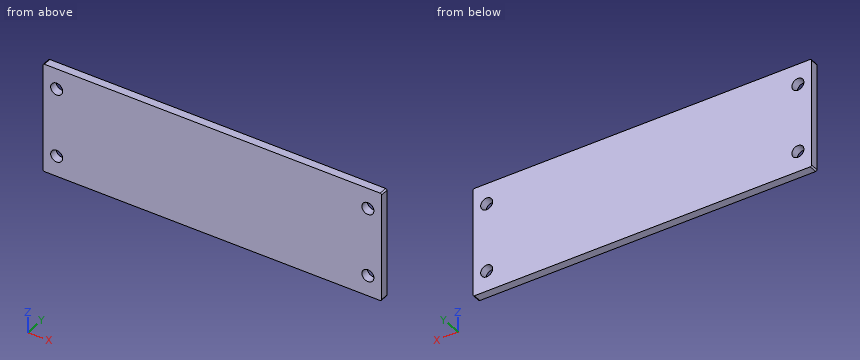
Autodesk Fusion 360 part; units mm, degrees
sketch "Sketch1" plane through (0, 0, 0) normal (0, 1, 0) x (1, 0, 0)
  line L0 (-61.5, -20) -> (61.5, -20)
  line L1 (62, -19.5) -> (62, 19.5)
  line L2 (61.5, 20) -> (-61.5, 20)
  line L3 (-62, 19.5) -> (-62, -19.5)
  line L4 (-62, -20) -> (62, 20) construction
  line L5 (62, -20) -> (-62, 20) construction
  line L6 (62, 20) -> (57, 20)
  line L7 (57, 20) -> (57, 12.5) construction
  line L8 (57, 12.5) -> (62, 12.5) construction
  line L9 (62, 12.5) -> (62, 20)
  line L10 (62, -20) -> (57, -20)
  line L11 (57, -20) -> (57, -12.5) construction
  line L12 (57, -12.5) -> (62, -12.5) construction
  line L13 (62, -12.5) -> (62, -20)
  line L14 (-62, -20) -> (-57, -20)
  line L15 (-57, -20) -> (-57, -12.5) construction
  line L16 (-57, -12.5) -> (-62, -12.5) construction
  line L17 (-62, -12.5) -> (-62, -20)
  line L18 (-62, 20) -> (-57, 20)
  line L19 (-57, 20) -> (-57, 12.5) construction
  line L20 (-57, 12.5) -> (-62, 12.5) construction
  line L21 (-62, 12.5) -> (-62, 20)
  circle A0 centre (57, -12.5) radius 2.2
  circle A1 centre (-57, -12.5) radius 2.2
  circle A2 centre (57, 12.5) radius 2.2
  circle A3 centre (-57, 12.5) radius 2.2
  arc A4 (61.5, -20) -> (62, -19.5) centre (61.5, -19.5) ccw
  arc A5 (-62, -19.5) -> (-61.5, -20) centre (-61.5, -19.5) ccw
  arc A6 (-61.5, 20) -> (-62, 19.5) centre (-61.5, 19.5) ccw
  arc A7 (62, 19.5) -> (61.5, 20) centre (61.5, 19.5) ccw
  dimension "d1" = 124
  dimension "d2" = 40
  dimension "d3" = 5
  dimension "d4" = 7.5
  dimension "d5" = 5
  dimension "d6" = 7.5
  dimension "d7" = 5
  dimension "d8" = 7.5
  dimension "d9" = 5
  dimension "d10" = 7.5
  dimension "d11" = 4.4
  dimension "d12" = 4.4
  dimension "d13" = 4.4
  dimension "d14" = 4.4
  dimension "d15" = 0.5
extrude "Extrude1" add sketch "Sketch1" along normal blind 3 contours L0 L1 L2 L3 L6 L9 L10 L13 L14 L17 L18 L21 A4 A5 A6 A7
For this review, take the finished solid that the model builds, in its own axes (mm). Give positions to 0.01 mm unless a question says otherwise; leave off trailing zeros. Loops run counter-clockwise (first coordinate to the right, second up) from the corner with the lowest first, then second, coordinate; pieces in that order, holes last. Notation, with made-up numbers: M -34,18.25 L 3,18.25 A24 cw 3,44.25 Z; hole C 0.25,39 d8. An arc over 180 degrees is marked long. Answer as a JSON object with one key per item and string values. Group by question number.
Q1. Add section A-A on x = 57. Give the boundary of the cut face in (y, z), and give its area (3 significant figures).
Q2. For probe 1 along X at (y, z) = (1.85, -12.5); probe 2 along Z at (x, y) = (-57, 2.05); probe 3 along X at (y, z) = (0.1, 13), list the stretches that pass through material, from the lowest coordinate up. Write a range as [from, to].
Q3. Add section B-B on z = -12.5. Give the boundary of the cut face in (x, y), and give its area (3 significant figures).
Checked values:
{
 "1": {"outline": "M 0,-20 L 3,-20 L 3,-14.7 L 0,-14.7 Z; M 0,-10.3 L 3,-10.3 L 3,10.3 L 0,10.3 Z; M 0,14.7 L 3,14.7 L 3,20 L 0,20 Z", "area": "93.6 mm²"},
 "2": {"probe 1": "[-62, -59.2], [-54.8, 54.8], [59.2, 62]", "probe 2": "[-20, -14.7], [-10.3, 10.3], [14.7, 20]", "probe 3": "[-62, -59.14], [-54.86, 54.86], [59.14, 62]"},
 "3": {"outline": "M -62,0 L -59.2,0 L -59.2,3 L -62,3 Z; M -54.8,0 L 54.8,0 L 54.8,3 L -54.8,3 Z; M 59.2,0 L 62,0 L 62,3 L 59.2,3 Z", "area": "346 mm²"}
}
